from build123d import *

# Parameters (mm, degrees)
F0_W          = 153
F0_H          = 99
F0_R          = 4
F1_DEPTH      = 20
F2_T          = -3
F3_R          = 4
F4_DEPTH      = 5
F5_R          = 1.6
F6_DEPTH      = 4
F7_R          = 1
F8_W          = 153
F8_H          = 8
F8_H_2        = 12
F9_DEPTH      = 3
F9_DEPTH_BACK = 2
F10_R         = 5
F11_W         = 13
F11_H         = 11.5
F12_DEPTH     = 3
F14_W         = 76
F14_H         = 10
F15_DEPTH     = 3
F17_D         = 5
F17_DEPTH     = 6
F17_TIP       = 1.5021515476


with BuildPart() as f1:
    # F0 (on Top) → F1 (new body)
    with BuildSketch(Plane.XY):
        with Locations((0, -2.5)):
            Rectangle(F0_W, F0_H)
        with Locations((-67.75, -38)):
            Circle(F0_R, mode=Mode.SUBTRACT)
        with Locations((67.75, -38)):
            Circle(F0_R, mode=Mode.SUBTRACT)
        with Locations((-67.75, 38)):
            Circle(F0_R, mode=Mode.SUBTRACT)
        with Locations((67.75, 38)):
            Circle(F0_R, mode=Mode.SUBTRACT)
        with Locations((-67.75, 38)):
            Circle(F0_R)
        with Locations((-67.75, -38)):
            Circle(F0_R)
        with Locations((67.75, -38)):
            Circle(F0_R)
        with Locations((67.75, 38)):
            Circle(F0_R)
    extrude(amount=F1_DEPTH)

    # F2
    f2_openings = [f1.faces().sort_by_distance(p)[0] for p in [
        (0, -2.5, 20),
    ]]
    offset(amount=F2_T, openings=f2_openings)

    # F3 (on face) → F4 (join)
    with BuildSketch(Plane.XY.offset(3)):
        with Locations((-67.75, 38)):
            Circle(F3_R)
        with Locations((-67.75, -38)):
            Circle(F3_R)
        with Locations((67.75, 38)):
            Circle(F3_R)
        with Locations((67.75, -38)):
            Circle(F3_R)
    extrude(amount=F4_DEPTH)

    # F5 (on face) → F6 (join)
    with BuildSketch(Plane.XY.offset(8)):
        with Locations((-67.75, -38)):
            Circle(F5_R)
        with Locations((-67.75, 38)):
            Circle(F5_R)
        with Locations((67.75, 38)):
            Circle(F5_R)
        with Locations((67.75, -38)):
            Circle(F5_R)
    extrude(amount=F6_DEPTH)

    # F7
    f7_edges = [f1.edges().sort_by_distance(p)[0] for p in [
        (-69.35, 38, 12),
        (-69.35, -38, 12),
        (66.15, 38, 12),
        (66.15, -38, 12),
    ]]
    fillet(f7_edges, radius=F7_R)

    # F8 (on face) → F9 (join, two sides)
    with BuildSketch(Plane.XZ.offset(52)) as f9_sk:
        Polygon((96.5, 32), (-96.5, 32), (-96.5, 12), (-76.5, 12), (-76.5, 20), (76.5, 20), (76.5, 12), (96.5, 12), align=None)
        with Locations((0, 16)):
            Rectangle(F8_W, F8_H)
        with Locations((0, 6)):
            Rectangle(F8_W, F8_H_2)
    extrude(amount=-F9_DEPTH)
    extrude(f9_sk.sketch, amount=F9_DEPTH_BACK)

    # F10
    f10_edges = [f1.edges().sort_by_distance(p)[0] for p in [
        (-96.5, -51.5, 32),
        (-96.5, -51.5, 12),
        (96.5, -51.5, 32),
        (96.5, -51.5, 12),
    ]]
    fillet(f10_edges, radius=F10_R)

    # F11 (on face) → F12 (cut, through all)
    with BuildSketch(Plane(origin=(0, 47, 0), x_dir=(-1, 0, 0), z_dir=(0, 1, 0))):
        with Locations((-44.25, 14.25)):
            Rectangle(F11_W, F11_H)
    extrude(amount=-F12_DEPTH, mode=Mode.SUBTRACT)

    # F14 (on face) → F15 (cut, through all)
    with BuildSketch(Plane.YZ.offset(76.5)):
        with Locations((0, 15)):
            Rectangle(F14_W, F14_H)
    extrude(amount=-F15_DEPTH, mode=Mode.SUBTRACT)

    # F17
    with Locations(Plane.XZ.offset(54)):
        with Locations((-86.5, 22), (0, 22), (86.5, 22)):
            Hole(F17_D / 2, depth=F17_DEPTH)
            with Locations((0, 0, -(F17_DEPTH + F17_TIP / 2))):  # 118° drill point
                Cone(0, F17_D / 2, F17_TIP, mode=Mode.SUBTRACT)


solid = f1.part
Geometry: final body of the model. Coordinates: model frame, mm. A direction names the side the tool comes from. Coordinates: 2 decimals unless noted, no trailing zeros. Loops run counter-clockwise (first coordinate to the right, second up) from the corner with the lowest first, then second, coordinate; pieces in that order, holes last. Notation, with made-up numbers: (7.5, 74) - (51.5, 74) arc R14 cw to (51.5, 86) - close; hole circle Ø9 at (45, -10.75). An arc over 180 degrees is marked (long way). Put each result on its own line as item: value. Start each with the question number.
Q1. Cut plane C-C, the plane z = 6. Return loops of the section in (x, y).
Q2. Line query: line 1 (X direction, y = 15.5, z = 5); line 2 (Y direction, x = -53, z = 12.5); line 3 (Z direction, x = 0, y = -50). Output: solid intervals per line, ascending.
Q3. Cut plane A-A, the plane z = 22. Return loops of the section in (x, y).
Q4. Set-up query: faces 1 (the flat face through (-66, 38, 8)), 2 (the flat face through (-84, -51, 12)), 3 (the cylindrical face through (-85, -51, 24)), 4 (the flat face through (-45, 45, 20)). Return all of +Z, -Z, +X, -X, +Y, -Y with unobstructed straight access to the full face (end or side cutting, diameter ignored); none if empty.
Q5. Cut plane B-B, the plane x = 0. Return loops of the section in (y, z), and give its area (3 significant figures).
Q6. Cut plane D-D, the plane y = 8.5. Return loops of the section in (x, z).
Q7. Pull-direction query (X, two-part tool) for faces 5 (the flat face through (66, 45, 20)), 6 (the cylindrical face through (-95, -51.54, 13.43)), 7 (the flat face through (-1, -49, 18)); classes: released by +X, released by -X, zero draft, split by the parting line, or undercut.
Q8. Pin query (flat end, axial travel): pin 1 Ø8 at (y, z) = (23.5, 11.5) entering from +X; pin 2 Ø0.9 at (x, y) = (74.5, -42) entering from +Z; pin 3 Ø1 at (x, y) = (68, 38) entering from +Z; pin 4 Ø4.5 at (x, z) = (86.5, 22) entering from -Y. Return the tip coordinate at first contact, or that it passes through.
Filled sheet:
1. outline: (-76.5, -54) - (76.5, -54) - (76.5, 47) - (-76.5, 47) - close; circle Ø8 at (-67.75, -38); circle Ø8 at (-67.75, 38); circle Ø8 at (67.75, -38); circle Ø8 at (67.75, 38); hole (-73.5, -49) - (73.5, -49) - (73.5, 44) - (-73.5, 44) - close
2. line 1: -76.5 to -73.5, 73.5 to 76.5
2. line 2: -54 to -49, 44 to 47
2. line 3: 0 to 19.5, 24.5 to 32
3. outline: (-96.5, -54) - (-89, -54) - (-89, -49) - (-96.5, -49) - close; (-84, -54) - (-2.5, -54) - (-2.5, -49) - (-84, -49) - close; (2.5, -54) - (84, -54) - (84, -49) - (2.5, -49) - close; (89, -54) - (96.5, -54) - (96.5, -49) - (89, -49) - close
4. face 1: +Z
4. face 2: -Z, -X, +Y, -Y
4. face 3: +Y, -Y
4. face 4: +Z, +X, -X, +Y
5. outline: (-54, 0) - (47, 0) - (47, 20) - (44, 20) - (44, 3) - (-49, 3) - (-49, 19.5) - (-54, 19.5) - close; (-54, 24.5) - (-49, 24.5) - (-49, 32) - (-54, 32) - close
5. area: 474 mm²
6. outline: (-76.5, 0) - (76.5, 0) - (76.5, 10) - (73.5, 10) - (73.5, 3) - (-73.5, 3) - (-73.5, 20) - (-76.5, 20) - close
7. face 5: zero draft
7. face 6: released by -X
7. face 7: undercut
8. pin 1: x = 76.5
8. pin 2: z = 20
8. pin 3: z = 12
8. pin 4: through
